Could you check a few things on this model? Use its own coordinates, in mm. A direction names the side the tool comes from. Give positions to 0.01 mm unless a question says otherwise; leave off trailing zeros. Order: outer loops, then holes, each group sorted by start corner. A loop starts at its lowest first (then second) coordinate and runs counter-clockwise, first axis right, second up. Notation, with made-up numbers: (49, 28) - (94, 28) arc R27 cw to (94, 45) - close; hole circle Ø4 at (-38, 20.5). An arc over 180 degrees is marked (long way). Put each result on its own line as item: value.
from build123d import *

# Parameters (mm, degrees)
EXTRUDE1_DEPTH = 5


with BuildPart() as part:
    # Sketch1 → Revolve1 (revolve)
    with BuildSketch(Plane.XY, mode=Mode.PRIVATE) as revolve1_sk:
        Polygon((0, 35.11626506), (4.5, 35.11626506), (2.5, 33.11626506), (2.5, 15.11626506), (0, 15.11626506), align=None)
    revolve(revolve1_sk.sketch.rotate(Axis((0, 45.521084337, 0), (0, -1, 0)), 90), axis=Axis((0, 45.521084337, 0), (0, -1, 0)))

    # Sketch2 → Extrude1 (cut, symmetric)
    with BuildSketch(Plane(origin=(0, 0, 0), x_dir=(0, 0, -1), z_dir=(1, 0, 0))):
        Polygon((-0.75, 35.11626506), (0, 33.61626506), (0.75, 35.11626506), align=None)
    extrude(amount=EXTRUDE1_DEPTH, both=True, mode=Mode.SUBTRACT)


solid = part.part
1) I'm going to push flat-ended pins straight in: pin 1 (4 mm diameter, centred on x = 1.5, y = 26.5, fed in from +Z); pin 2 (3 mm diameter, centred on x = 0, y = 21, fed in from -Z); pin 3 (4 mm diameter, centred on y = 31, z = 3, fed in from +X). Where does each tip first touch, or does it pass through?
Filled in:
pin 1: stops at z = 2.5
pin 2: stops at z = -2.5
pin 3: stops at x = 2.29
2) Suppose I cut it at A-A, the plane x = 0. List the corners of the cut face in (y, z) for me.
Filled in:
outline: (15.12, -2.5) - (33.12, -2.5) - (35.12, -4.5) - (35.12, -0.75) - (33.62, 0) - (35.12, 0.75) - (35.12, 4.5) - (33.12, 2.5) - (15.12, 2.5) - close
3) If I drill on line 1 (Y direction, x = -1.25, z = -3.25); line 2 (Y direction, x = 3.25, z = 2.5); line 3 (X direction, y = 30.5, z = -1.75), over which ranges is the centre line in solid material (lowest first)? Write a range as [from, to].
Filled in:
line 1: y = [34.1, 35.12]
line 2: y = [34.72, 35.12]
line 3: x = [-1.79, 1.79]
4) Which directions (+Z, -Z, +X, -X, +Y, -Y) give clear straight access to the entire face, cutting with the end or side of a thin tool? Please do faces 1 (the flat face through (0, 15.116, 0)), 2 (the cylindrical face through (-0.1, 24, -2.5)).
Filled in:
face 1: +Z, -Z, +X, -X, -Y
face 2: -Y
5) Suppose I cut it at B-B, the plane y = 25.25. List the corners of the cut face in (x, z) for me.
Filled in:
outline: circle Ø5 at (0, 0)
